from build123d import *

# Parameters (mm, degrees)
PAD_DEPTH    = 5
PAD001_DEPTH = 30
SKETCH002_R  = 12.9
POCKET_DEPTH = 34.3976445385


with BuildPart() as part:
    # Sketch → Pad (new body)
    with BuildSketch(Plane.XY):
        with BuildLine():
            Line((33.5410196625, 30), (50, 30))
            Line((50, 30), (50, 60))
            Line((0, 60), (50, 60))
            ThreePointArc((0, 60), (-10.1461187235, 59.1359135792), (-20, 56.5685424949))
            Line((-20, 40.3112887415), (-20, 56.5685424949))
            ThreePointArc((33.5410196625, 30), (8.5100218715, 44.1880020792), (-20, 40.3112887415))
        make_face()
    extrude(amount=PAD_DEPTH)

    # Sketch001 → Pad001 (new body)
    with BuildSketch(Plane.XY.offset(5)):
        Polygon((-0.4786107292, 60), (33.9483604854, 49.47461863), (30.4399000287, 37.9989615584), (-3.9870711859, 48.5243429284), align=None)
    extrude(amount=PAD001_DEPTH)

    # Sketch002 → Pocket (cut, through all)
    with BuildSketch(Plane(origin=(16.7348748781, 54.737309315, 0), x_dir=(-0.956304756, 0.2923717047, 0), z_dir=(0.2923717047, 0.956304756, 0))):
        with Locations((0, 35)):
            Circle(SKETCH002_R)
    extrude(amount=-POCKET_DEPTH, mode=Mode.SUBTRACT)


solid = part.part
Read the model definition and answer for the solid it produces. Units are mm, in the model's axes. A direction names the side the tool comes from. Give positions to 0.01 mm unless a question says otherwise; leave off trailing zeros. Write each loop counter-clockwise with the first axis right and the second up, starting at its lowest first coordinate (ties: lowest second). Pieces come first, ordered by that corner, then holes. Notation, with made-up numbers: (53.25, 0.25) -> (80.25, 0.25) arc R35 ccw to (80.25, 37.25) -> close; hole circle Ø7 at (-38, -9). An arc over 180 degrees is marked (long way). Answer as a JSON object with one key per item and string values. Group by question number.
1) A tool of negligible diameter and unlimited length cuts with its end or side. For faces 1 (the flat face through (32.22, 43.82, 19.79)), 2 (the flat face through (16.494, 54.811, 16.457)), 3 (the flat face through (-2.26, 54.18, 19.79)), 4 (the flat face through (13.467, 43.188, 16.457)), from which of +Z, -Z, +X, -X, +Y, -Y can it reach the whole face along a straight path? Write none if from no direction.
2) Each of these flat-tipped pins is pushed along its axis until it touches: P1, Ø10, axis at y = 52.5, z = 31, coming from the -X side; P2, Ø12, axis at x = 19, z = 18.5, coming from the -Y side; P3, Ø5, axis at x = 31, z = 17.5, coming from the -Y side. Where does it stop, or does it pass through?
3) Find section A-A (z = 30.5). Write down the section's boundary in (x, y).
4) Consider L1, parallel to Z at x = 42, y = 57; L2, parallel to X at y = 33, z = 4; L3, parallel to Y at x = 5.5, z = 22. Determine where each line is inside the solid, lowest interval first. Write a range as from..to.
5) Find section C-C (x = -14.5). Write down the section's boundary in (y, z), and give its area (3 significant figures).
6) Find section D-D (z = 26). Write down the section's boundary in (x, y), and give its area (3 significant figures).
7) Find section B-B (z = 2). Write down the section's boundary in (x, y).
8) The mould has two halves that part along X. Classify faces 5 (the flat face through (-20, 48, 2)), 6 (the flat face through (22, 55, 5)), 7 (the cylindrical face through (8.91, 44.11, 2.46)): +X half, -X half, draft (parallel to the pull), parting line (faces both ways), or undercut.
Values follow:
{
 "1": {"face 1": "+Z, +X, -Y", "face 2": "+Z, +X, +Y", "face 3": "+Z, -X, +Y", "face 4": "+Z, -X, -Y"},
 "2": {"P1": "stops at x = -3.99", "P2": "stops at y = 39.66", "P3": "stops at y = 38"},
 "3": {"outline": "(-3.99, 48.52) -> (1.67, 46.8) -> (5.17, 58.27) -> (-0.48, 60) -> close; (24.79, 39.73) -> (30.44, 38) -> (33.95, 49.47) -> (28.3, 51.2) -> close"},
 "4": {"L1": "z = 0..5", "L2": "x = 30.59..50", "L3": "y = 45.62..58.17"},
 "5": {"outline": "(42.6, 0) -> (58.22, 0) -> (58.22, 5) -> (42.6, 5) -> close", "area": "78.1 mm2"},
 "6": {"outline": "(-3.99, 48.52) -> (4.39, 45.96) -> (7.9, 57.44) -> (-0.48, 60) -> close; (22.06, 40.56) -> (30.44, 38) -> (33.95, 49.47) -> (25.57, 52.04) -> close", "area": "210 mm2"},
 "7": {"outline": "(-20, 40.31) arc R45 cw to (33.54, 30) -> (50, 30) -> (50, 60) -> (0, 60) arc R60 ccw to (-20, 56.57) -> close"},
 "8": {"face 5": "-X half", "face 6": "draft", "face 7": "undercut"}
}
